Geometry: final body of the model. Coordinates: model frame, mm. A direction names the side the tool comes from. Round coordinates to 2 decimals unless told otherwise and drop trailing zeros. Order: outer loops, then holes, each group sorted by start corner. A loop starts at its lowest first (then second) coordinate and runs counter-clockwise, first axis right, second up. Notation, with made-up numbers: M 12.5,-34.5 L 54.5,-34.5 A14 cw 54.5,-28.5 Z; hole C -36,87.5 d6. An arc over 180 degrees is marked long. Return JSON: item names as keys, results as strings. Group by question number.
Q1. Cut plane A-A on z = -49. Output: boundary loops of the cut face in (x, y), and give its area (3 significant figures).
Q2. Cut plane D-D on x = 20. Output: boundary loops of the cut face in (y, z), and give its area (3 significant figures).
Q3. Access query for faces 4 (the face through (0, 2, -0.9)), 5 (the face through (0, -5, 0)), 6 (the face through (19, 0, -48)). Directions: +Z, -Z, +X, -X, +Y, -Y. A direction counts if a zero-diameter tool reaches every point of the face in a straight line with its end or side. Return the directions, or none.
Q4. Cut plane C-C on z = -9. Output: boundary loops of the cut face in (x, y).
Q5. Ray query, probe 1 along Z at (x, y) = (14, -14.5); probe 2 along Z at (x, y) = (-5, 11.5); probe 3 along Y at (x, z) = (-8, -6). Return the intervals inside material, ascending.
Q6. Cut plane B-B on x = -17. Output: boundary loops of the cut face in (y, z).
Q7. Contact query for flat-ended pins moving along their axis: pin 1 (5 mm diameter, centred on x = 6.5, y = 7.5, fed in from -Z); pin 2 (1.5 mm diameter, centred on x = 20, y = -18.5, fed in from +Z); pin 3 (6 mm diameter, centred on y = -3.5, z = -41.5, fed in from +X). Output: stop coordinate, or through.
Q8. Mould query, pull axis X, two halves, no side actions, for faces 1 (the face through (23.846, 7.509, -4.93)), 2 (the face through (-15.6, 1.8, -48.5)), 3 (the face through (-18, 0, -88)). Classes: released by +X, released by -X, zero draft, split by the parting line, or undercut.
Autodesk Inventor part; units mm, degrees
ref_plane "YZ Plane" through (0, 0, 0) normal (1, 0, 0) x (0, 1, 0)
ref_plane "XZ Plane" through (0, 0, 0) normal (0, 1, 0) x (-1, 0, 0)
ref_plane "XY Plane" through (0, 0, 0) normal (0, 0, 1) x (1, 0, 0)
sketch "Sketch1" plane through (0, 0, 0) normal (0, 0, 1) x (1, 0, 0)
  circle A0 centre (0, 0) radius 25
  line L0 (9.0545, 19) -> (-15.9277, 6.5172) construction
  line L1 (-15.9277, 6.5172) -> (4.4593, -0.1187) construction
  line L2 (4.4593, -0.1187) -> (8.9648, -0.1187) construction
  line L3 (8.9648, -0.1187) -> (-5.7342, -19.5656) construction
  line L4 (-5.7342, -19.5656) -> (-5.7342, -19.5656) construction
  spline S0 degree 4 poles (9.0545, 19) (-15.9277, 6.5172) (4.4593, -0.1187) (8.9648, -0.1187) (-5.7195, -19.5462) (-5.7342, -19.5656) knots 1 1 1 1 1 2 3 3 3 3 3
  line L5 (9.0545, 19) -> (1.8467, 5.2615) construction
  line L6 (1.8467, 5.2615) -> (8.9648, -0.1187) construction
  line L7 (8.9648, -0.1187) -> (9.0545, 0) construction
  line L8 (9.0545, 0) -> (4.4598, -12) construction
  line L9 (4.4598, -12) -> (-5.7342, -19.5656) construction
  spline S1 degree 4 poles (9.0545, 19) (1.8467, 5.2615) (8.9648, -0.1187) (9.0545, 0) (4.4598, -12) (-5.7342, -19.5656) knots 1 1 1 1 1 2 3 3 3 3 3
extrude "Extrusion1" add sketch "Sketch1" against normal blind 10 contours A0 | S1 S0
sketch "Sketch2" plane through (0, 0, 0) normal (0, 0, 1) x (1, 0, 0)
  line L0 (4, 18) -> (-23, 7) construction
  line L1 (-23, 7) -> (4, -3) construction
  spline S0 degree 2 poles (4, 18) (-23, 7) (4, -3) knots 1 1 1 2 2 2
  line L2 (4, -3) -> (15.0435, -8.5217) construction
  line L3 (15.0435, -8.5217) -> (-7, -17) construction
  line L4 (-7, -17) -> (-7.0477, -17) construction
  spline S1 degree 3 poles (4, -3) (15.0435, -8.5217) (-7, -17) (-7.0477, -17) knots 1 1 1 1 2 2 2 2
  line L5 (4, 18) -> (-12, 4) construction
  line L6 (-12, 4) -> (9.5217, -1) construction
  spline S2 degree 2 poles (4, 18) (-12, 4) (9.5217, -1) knots 1 1 1 2 2 2
  line L7 (9.5217, -1) -> (14.1934, -13.1463) construction
  line L8 (14.1934, -13.1463) -> (-7.0477, -17) construction
  spline S3 degree 2 poles (9.5217, -1) (14.1934, -13.1463) (-7.0477, -17) knots 1 1 1 2 2 2
  point P0 (0, 0)
extrude "Extrusion2" cut sketch "Sketch2" against normal blind 0.9
sketch "Sketch3" plane through (0, 0, -10) normal (0, 0, -1) x (-1, 0, 0)
  circle A0 centre (-16, 0) radius 3
  circle A1 centre (18, 0) radius 3
  point P0 (0, 0)
extrude "Extrusion3" add sketch "Sketch3" along normal blind 78
properties part number "Photoresistor"
Result sheet:
{
 "1": {"outline": "C -18,0 d6; C 16,0 d6", "area": "56.5 mm²"},
 "2": {"outline": "M -15,-10 L 15,-10 L 15,0 L -15,0 Z", "area": "300 mm²"},
 "3": {"face 4": "+Z", "face 5": "+Z, +X, -X, +Y, -Y", "face 6": "-Z"},
 "4": {"outline": "C 0,0 d50"},
 "5": {"probe 1": "z = -10 to 0", "probe 2": "z = -10 to -0.9", "probe 3": "y = -23.69 to 23.69"},
 "6": {"outline": "M -18.33,-10 L -2.83,-10 L -2.83,-88 L 2.83,-88 L 2.83,-10 L 18.33,-10 L 18.33,0 L -18.33,0 Z"},
 "7": {"pin 1": "stops at z = -10", "pin 2": "passes through", "pin 3": "stops at x = 18.96"},
 "8": {"face 1": "split by the parting line", "face 2": "undercut", "face 3": "zero draft"}
}
